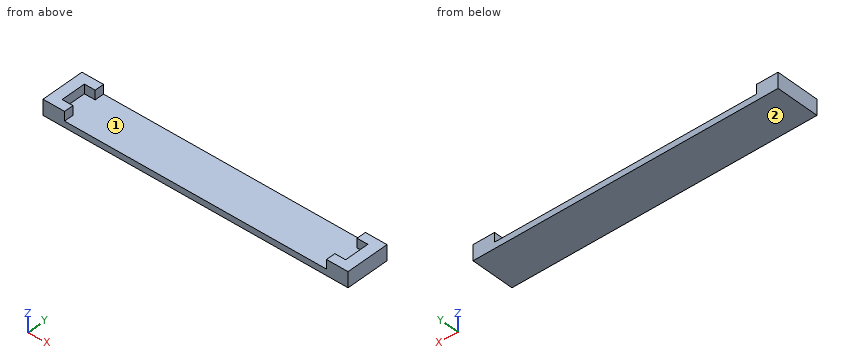
```python
from build123d import *

# Parameters (mm, degrees)
F1_DEPTH = 2
F2_DEPTH = 5
F3_DEPTH = 5


with BuildPart() as f1:
    # F0 (on Top) → F1 (new body)
    with BuildSketch(Plane.XY):
        Polygon((42.5, 4), (42.5, 7), (-42.5, 7), (-42.5, 4), (-46, 4), (-46, -4), (-42.5, -4), (-42.5, -7), (42.5, -7), (42.5, -4), (46, -4), (46, 4), align=None)
    extrude(amount=F1_DEPTH)

    # F0 (on Top) → F2 (join)
    with BuildSketch(Plane.XY):
        Polygon((-42.5, 4), (-42.5, 7), (-49.5, 7), (-49.5, -7), (-42.5, -7), (-42.5, -4), (-46, -4), (-46, 4), align=None)
    extrude(amount=F2_DEPTH)

    # F0 (on Top) → F3 (join)
    with BuildSketch(Plane.XY):
        Polygon((49.5, -7), (49.5, 7), (42.5, 7), (42.5, 4), (46, 4), (46, -4), (42.5, -4), (42.5, -7), align=None)
    extrude(amount=F3_DEPTH)


solid = f1.part
```
Build history of the part. All positions in model axes, mm. Face numbers are marked on the shaded views. Round coordinates to 2 decimals unless told otherwise and drop trailing zeros. Write each loop counter-clockwise with the first axis right and the second up, starting at its lowest first coordinate (ties: lowest second). Pieces come first, ordered by that corner, then holes. Notation, with made-up numbers: (11, 79.5) - (69, 79.5) arc R24 ccw to (69, 98.5) - close; hole circle Ø3 at (89.5, 59). An arc over 180 degrees is marked (long way). Write each question's results on one line, items separated by ' | '. Start each with the question number.
Item 1: Saw through at A-A (z = 3.1). Write the cut outline in (x, y).
Item 2: Saw through at C-C (x = 36.5). Write the cut outline in (y, z).
Item 3: Saw through at B-B (y = 5.5). Write the cut outline in (x, z), and give its area (3 significant figures).
Item 4: Drop a flat-ended pin along its axis: P1, Ø4, axis at x = -19, y = -1, coming from the +Z side. Give the stop position or say it passes through.
Item 5: Wall check: L1, parallel to X at y = 2, z = 2.45; L2, parallel to Z at x = 19.5, y = -3.25; L3, parallel to X at y = 6, z = 4.25. Give the ranges that are in metal, low to high. Write a range as [from, to].
Item 6: Mould opens along X. For the marked faces 1 and 2 say: pulls with the +X half, pulls with the -X half, needs draft (parallel to the pull), parting line crosses it, or undercut.
Results are:
1) outline: (-49.5, -7) - (-42.5, -7) - (-42.5, -4) - (-46, -4) - (-46, 4) - (-42.5, 4) - (-42.5, 7) - (-49.5, 7) - close; (42.5, -7) - (49.5, -7) - (49.5, 7) - (42.5, 7) - (42.5, 4) - (46, 4) - (46, -4) - (42.5, -4) - close
2) outline: (-7, 0) - (7, 0) - (7, 2) - (-7, 2) - close
3) outline: (-49.5, 0) - (49.5, 0) - (49.5, 5) - (42.5, 5) - (42.5, 2) - (-42.5, 2) - (-42.5, 5) - (-49.5, 5) - close | area: 240 mm²
4) P1: stops at z = 2
5) L1: x = [-49.5, -46], [46, 49.5] | L2: z = [0, 2] | L3: x = [-49.5, -42.5], [42.5, 49.5]
6) face 1: undercut | face 2: needs draft
